Input: part model. Units: mm. Frame: model coordinates. Face numbers are marked on the shaded views. Coordinates: 2 decimals unless noted, no trailing zeros. Write each loop counter-clockwise with the first axis right and the second up, starting at its lowest first coordinate (ties: lowest second). Pieces come first, ordered by that corner, then holes.
1) Line query: L1, parallel to Z at x = 1, y = -7; L2, parallel to Z at x = 7.75, y = 1.25; L3, parallel to X at y = -0.25, z = 33.5. Output: solid intervals per line, ascending.
2) Draft query along X for the marked faces 1, 2 and 3. Return one class per face: pulls with the +X half, pulls with the -X half, needs draft (parallel to the pull), parting line crosses it, or undercut.
3) Pin query (flat end, axial travel): pin 1 Ø1.5 at (x, y) = (-1, 4) entering from +Z; pin 2 Ø5 at (x, z) = (0, 24.5) entering from +Y; pin 3 Ø5 at (y, z) = (-4, 30) entering from +X; pin 4 Ø5 at (x, y) = (-1.5, 0) entering from +Z. Return the tip coordinate at first contact, or that it passes through.
4) Section query B-B (z = 37.5). Output: boundary loops of the cut face in (x, y).
5) Section query A-A (z = 42.5). Output: boundary loops of the cut face in (x, y), then the cut area to 3 significant figures.
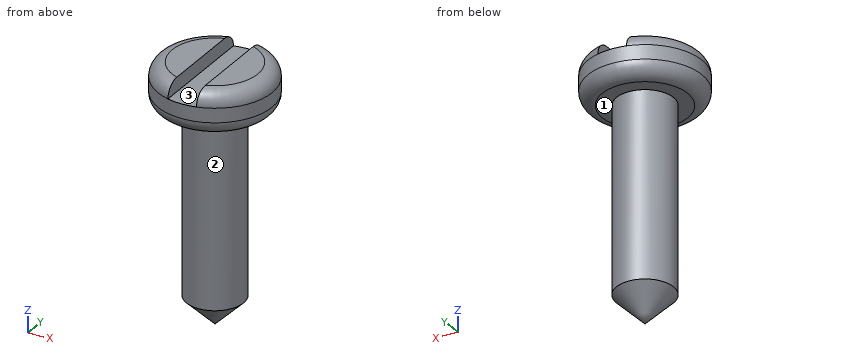
from build123d import *

# Parameters (mm, degrees)
F2_R     = 2.54
F3_W     = 5.08
F3_H     = 22.090304
F4_DEPTH = 2.54


with BuildPart() as f1:
    # F0 (on Front) → F1 (revolve)
    with BuildSketch(Plane.XZ):
        Polygon((0, 45.72), (0, 0), (5.08, 5.08), (5.08, 38.1), (10.16, 38.1), (10.16, 45.72), align=None)
    revolve(axis=Axis((0, 0, 22.86), (0, 0, 1)))

    # F2
    f2_edges = [f1.edges().sort_by_distance(p)[0] for p in [
        (-10.16, 0, 45.72),
        (-10.16, 0, 38.1),
    ]]
    fillet(f2_edges, radius=F2_R)

    # F3 (on face) → F4 (cut)
    with BuildSketch(Plane.XY.offset(45.72)):
        with Locations((0, -0.139493)):
            Rectangle(F3_W, F3_H)
    extrude(amount=-F4_DEPTH, mode=Mode.SUBTRACT)


solid = f1.part
Answer:
1. L1: z = 38.1 to 43.18
1. L2: z = 38.11 to 45.71
1. L3: x = -5.07 to 5.07
2. face 1: needs draft
2. face 2: parting line crosses it
2. face 3: undercut
3. pin 1: stops at z = 43.18
3. pin 2: stops at y = 5.08
3. pin 3: stops at x = 4.85
3. pin 4: stops at z = 45.72
4. outline: circle Ø10.16 at (0, 0)
5. outline: circle Ø20.32 at (0, 0)
5. area: 324 mm2
